Study the drawing (mm; zero at the part's minimum x, y, z) and answer. Give positions to 0.01 mm unless a question says otherwise; leave off trailing zeros. Loops run counter-clockwise (first coordinate to the right, second up) from the corner with the lowest first, then second, coordinate; pieces in that order, holes last. Notation, with made-up numbers: (-19.75, -15) - (-3.75, -15) arc R18 ccw to (-3.75, 20) - close; hole circle Ø10 at (41, 29). An arc over 180 degrees is marked (long way). Answer in a Markdown table with one row per item. Add a question column.
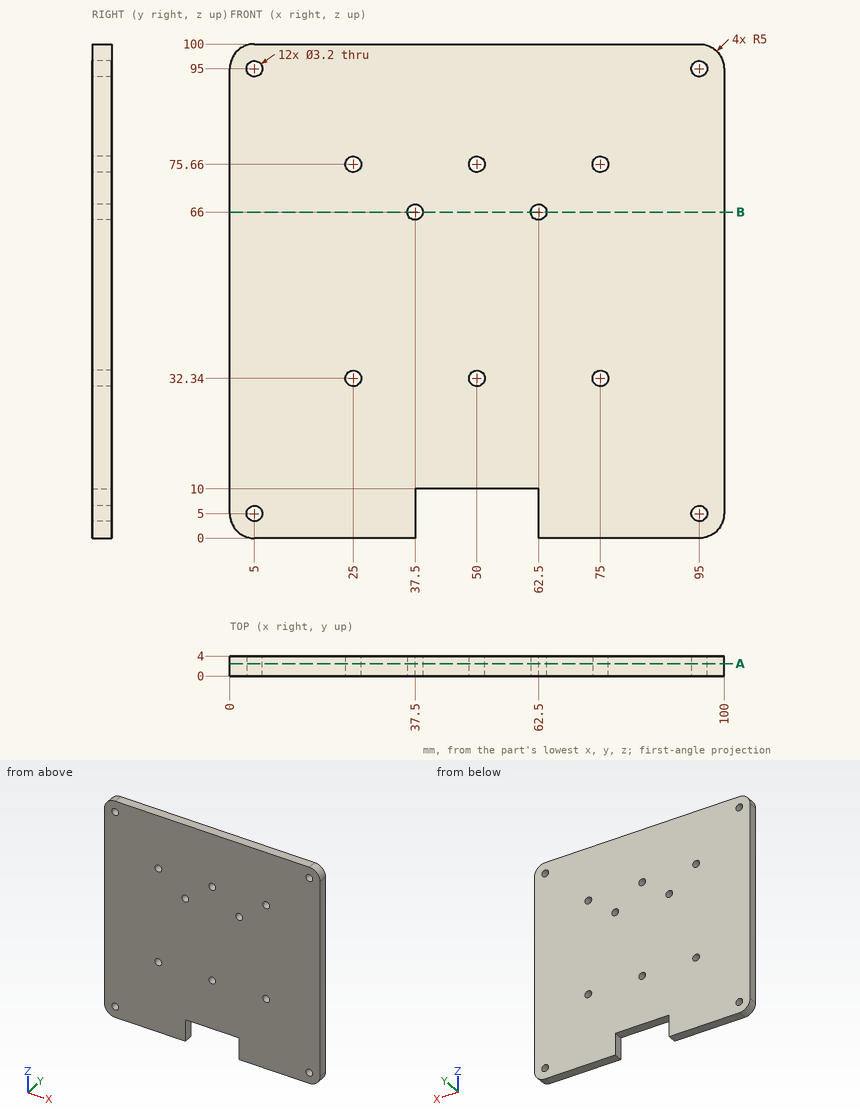
(1) Given pin 1 Ø2 at (y, z) = (1.5, 3) entering from +X; pin 2 Ø1.9 at (x, z) = (5, 5) entering from -Y; pin 3 Ø1.2 at (y, z) = (1.5, 3) entering from -X, each flat-ended and moving along its own axis, determine where each tip first touches the part or whether it passes through.
(2) Find the intervals of material crossed by line 1 along X through (y, z) = (1.1, 32.34); line 2 along X through (y, z) = (1.3, 5); line 3 along Z through (x, y) = (5, 1.8), in increasing order. Write a range as [from, to].
(3) A cutting plane is placed at B-B on z = 66. Determine the outline of the cut face in (x, y).
(4) A cutting plane is placed at A-A on y = 2.5. Give the number of separate pieces and of enclosed holes in the cut face, plus the area to 3 significant figures.
Evaluation:
| question | item | result |
|---|---|---|
| 1 | pin 1 | stops at x = 99.9 |
| 1 | pin 2 | passes through |
| 1 | pin 3 | stops at x = 0.2 |
| 2 | line 1 | x = [0, 23.4], [26.6, 48.4], [51.6, 73.4], [76.6, 100] |
| 2 | line 2 | x = [0, 3.4], [6.6, 37.5], [62.5, 93.4], [96.6, 100] |
| 2 | line 3 | z = [0, 3.4], [6.6, 93.4], [96.6, 100] |
| 3 | outline | (0, 0) - (35.9, 0) - (35.9, 4) - (0, 4) - close; (39.1, 0) - (60.9, 0) - (60.9, 4) - (39.1, 4) - close; (64.1, 0) - (100, 0) - (100, 4) - (64.1, 4) - close |
| 4 | separate pieces | 1 |
| 4 | enclosed holes | 12 |
| 4 | area | 9,630 mm² |
